Geometry check sheet. Reference: drawing and pictorial views, mm from the part's lowest x, y, z. Give positions to 0.01 mm unless a question says otherwise; leave off trailing zeros. Put each result on its own line as item: value. Start each with the question number.
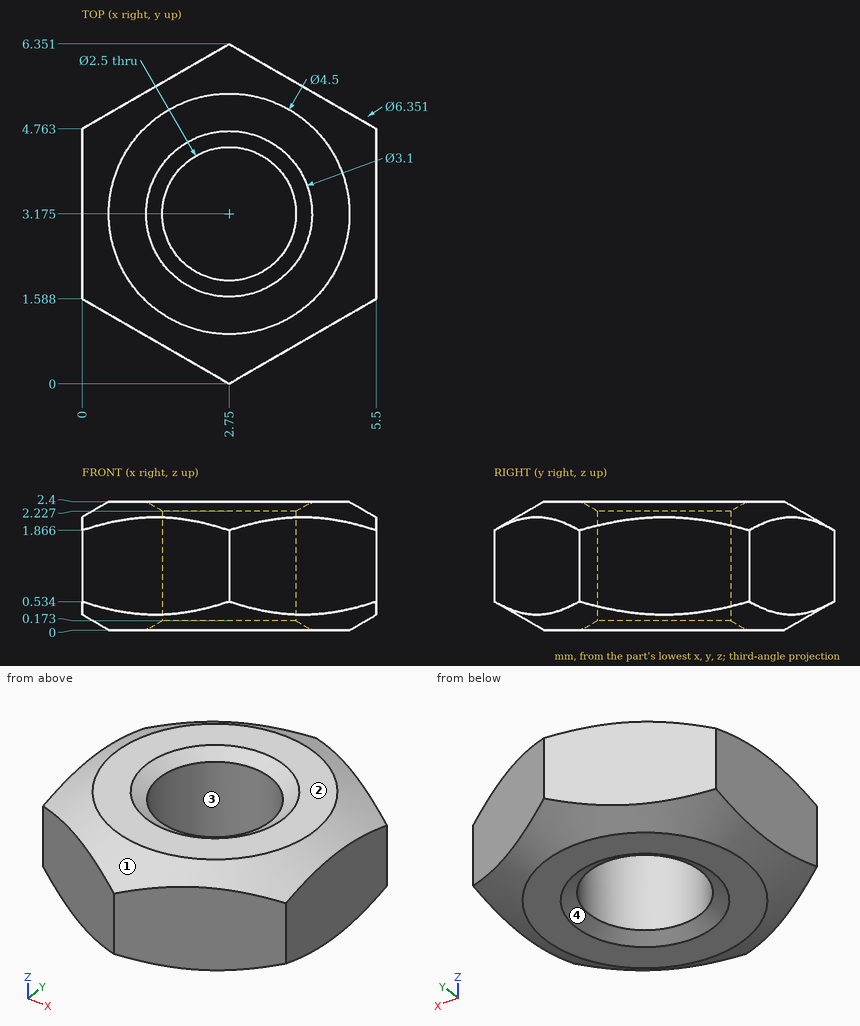
1) Draft check along Y on the marked faces 1, 2, 3 and 4. Enter one of: pulls with the +Y half, pulls with the -Y half, needs draft (parallel to the pull), parting line crosses it, or undercut.
2) Depth check by flat-ended pin: P1, Ø1, axis at x = 1, z = 2, coming from the +Y side; P2, Ø1.5, axis at x = 2.75, y = 3.18, coming from the -Z side. Enter the tip coordinate at first touch or a pass-through.
3) Scan lines: line 1 along Y through (x, z) = (2.25, 1.85); line 2 along Y through (x, z) = (2.1, 0.25) (1 decimal); line 3 along X through (y, z) = (4, 1.8). Record each from-to range of solid material in increasing order. Write a range as from..to.
Results are:
1. face 1: parting line crosses it
1. face 2: needs draft
1. face 3: undercut
1. face 4: undercut
2. P1: stops at y = 5.63
2. P2: passes through
3. line 1: y = 0.29..2.03, 4.32..6.06
3. line 2: y = 0.6..2.1, 4.2..5.8
3. line 3: x = 0..1.81, 3.69..5.5
